Read the model definition and answer for the solid it produces. Units are mm, in the model's axes. A direction names the side the tool comes from. Coordinates: 2 decimals unless noted, no trailing zeros. Order: outer loops, then holes, each group sorted by start corner. A loop starts at its lowest first (then second) coordinate and runs counter-clockwise, first axis right, second up. Notation, with made-up numbers: (-4, 56) -> (16, 56) arc R5 ccw to (16, 65) -> close; hole circle Ø7 at (-28, 30). An arc over 180 degrees is marked (long way). Answer as a JSON object with one key per item and string values. Group by question number.
1) Section A-A on z = 1.5 is taken. Determine the outline of the cut face in (x, y).
2) Given pin 1 (2 mm diameter, centred on x = -11.5, z = 0, fed in from -Y); pin 2 (4 mm diameter, centred on y = -13.5, z = 1.5, fed in from +X); pin 3 (5 mm diameter, centred on y = -12.5, z = 1.5, fed in from -X), each flat-ended and moving along its own axis, determine where each tip first touches the part or whether it passes through.
3) A tool of negligible diameter and unlimited length cuts with its end or side. For faces 4 (the cylindrical face through (-4.95, -22.27, 1.13)), 5 (the cylindrical face through (-11.06, 17.34, -1.5)), 6 (the flat face through (0, 0, -6.604)), from which of +Z, -Z, +X, -X, +Y, -Y can it reach the whole face along a straight path? Write none if from no direction.
4) Section B-B on z = -2.5 is taken. Determine the outline of the cut face in (x, y), and give its area (3 significant figures).
5) Consider L1, parallel to Z at x = 10, y = 19.5; L2, parallel to Z at x = -16, y = 15; L3, parallel to Y at x = -6, z = -5. Determine where each line is inside the solid, lowest interval first.
6) Determine the mould class of faces 1 (the cylindrical face through (-10.767, -20.379, -4.175)), 2 (the flat face through (0, 0, 3.556)), 3 (the flat face through (-12, 17, 0)) for opening direction Z: released by +Z, released by -Z, zero draft, split by the parting line, or undercut.
from build123d import *

# Parameters (mm, degrees)
SKETCH1_R           = 22.811957467
BOSS_EXTRUDE1_DEPTH = 3.556
SKETCH2_R           = 20.565315444
BOSS_EXTRUDE2_DEPTH = 3.048
SKETCH3_R           = 22.86
BOSS_EXTRUDE3_DEPTH = 3.556
FILLET2_R           = 1.27
FILLET3_R           = 1.27


with BuildPart() as part:
    # Sketch1 → Boss-Extrude1 (new body)
    with BuildSketch(Plane.XY):
        Circle(SKETCH1_R)
    extrude(amount=BOSS_EXTRUDE1_DEPTH)

    # Sketch2 → Boss-Extrude2 (add)
    with BuildSketch(Plane(origin=(0, 0, 0), x_dir=(-1, 0, 0), z_dir=(0, 0, -1))):
        Circle(SKETCH2_R)
    extrude(amount=BOSS_EXTRUDE2_DEPTH)

    # Sketch3 → Boss-Extrude3 (add)
    with BuildSketch(Plane(origin=(-3.118678077, -2.889960947, -3.048), x_dir=(-1, 0, 0), z_dir=(0, 0, -1))):
        with Locations((-2.900665776, 2.79149385)):
            Circle(SKETCH3_R)
    extrude(amount=BOSS_EXTRUDE3_DEPTH)

    # Fillet2
    fillet2_edges = [part.edges().sort_by_distance(p)[0] for p in [
        (-22.811957467, 0, 3.556),
    ]]
    fillet(fillet2_edges, radius=FILLET2_R)

    # Fillet3
    fillet3_edges = [part.edges().sort_by_distance(p)[0] for p in [
        (22.641987699, -0.098467097, -6.604),
    ]]
    fillet(fillet3_edges, radius=FILLET3_R)


solid = part.part
Worked answers:
{
 "1": {"outline": "circle Ø45.62 at (0, 0)"},
 "2": {"pin 1": "stops at y = -20.25", "pin 2": "stops at x = 19.7", "pin 3": "stops at x = -20.5"},
 "3": {"face 4": "+Z", "face 5": "none", "face 6": "-Z, +X, -X, +Y, -Y"},
 "4": {"outline": "circle Ø41.13 at (0, 0)", "area": "1,330 mm²"},
 "5": {"L1": "z = -6.5 to -3.05, 0 to 3.5", "L2": "z = -6.58 to -3.05, 0 to 3.49", "L3": "y = -22.22 to 22.02"},
 "6": {"face 1": "zero draft", "face 2": "released by +Z", "face 3": "undercut"}
}
